Study the drawing (mm; zero at the part's minimum x, y, z) and answer. A direction names the side the tool comes from. Coordinates: 2 decimals unless noted, no trailing zeros. Order: outer loops, then holes, each group sorted by start corner. A loop starts at its lowest first (then second) coordinate and runs counter-clockwise, first axis right, second up.
1. Flat-ended cylindrical pins translate along their axes: pin 1 Ø6 at (x, z) = (38.5, 38.5) entering from -Y; pin 2 Ø4 at (y, z) = (7.5, 5) entering from -X; pin 3 Ø1.2 at (x, z) = (51.5, 2.5) entering from +Y; pin 4 Ø1.6 at (x, y) = (3.35, 15.2) entering from -Z. Find the tip coordinate at first contact, or state that the pin passes through.
2. Find the intervals of material crossed by probe 1 along Y at (x, z) = (53.25, 27.7); probe 2 along Z at (x, y) = (51, 9.5); probe 3 along Z at (x, y) = (42.5, 15.5), in increasing order.
3. The part is cut by section D-D, the plane y = 5.8. Give the vertices of the cut face in (x, z).
4. The part is cut by section B-B, the plane z = 27.5. Give the vertices of the cut face in (x, y), then the cut area to 3 significant figures.
5. Determine the mould class of the marked faces 1, 2 and 3 for opening direction Z: +Z half, -Z half, draft (parallel to the pull), parting line (faces both ways), or undercut.
6. The part is cut by section A-A, the plane x = 50. Give the vertices of the cut face in (y, z), then the cut area to 3 significant figures.
7. The part is cut by section C-C, the plane x = 38.2. Give the vertices of the cut face in (y, z).
8. A tool of negligible diameter and unlimited length cuts with its end or side. For the marked faces 4, 5, 6 and 7, from which of +Z, -Z, +X, -X, +Y, -Y can it reach the whole face along a straight path? Write none if from no direction.
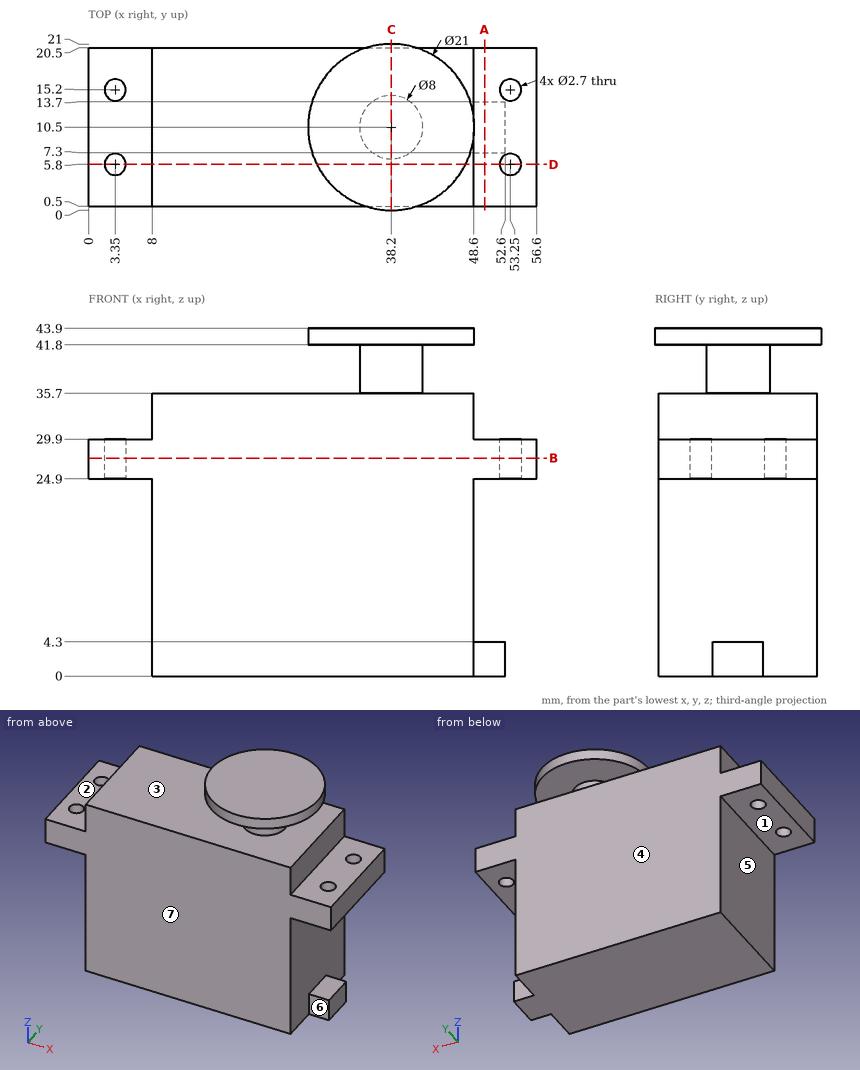
Geometry says:
1. pin 1: stops at y = 0.5
1. pin 2: stops at x = 8
1. pin 3: stops at y = 13.7
1. pin 4: passes through
2. probe 1: y = 0.5 to 4.45, 7.15 to 13.85, 16.55 to 20.5
2. probe 2: z = 0 to 4.3, 24.9 to 29.9
2. probe 3: z = 0 to 35.7, 41.8 to 43.9
3. outline: (0, 24.9) - (2, 24.9) - (2, 29.9) - (0, 29.9) - close; (4.7, 24.9) - (8, 24.9) - (8, 0) - (48.6, 0) - (48.6, 24.9) - (51.9, 24.9) - (51.9, 29.9) - (48.6, 29.9) - (48.6, 35.7) - (8, 35.7) - (8, 29.9) - (4.7, 29.9) - close; (28.81, 41.8) - (47.59, 41.8) - (47.59, 43.9) - (28.81, 43.9) - close; (54.6, 24.9) - (56.6, 24.9) - (56.6, 29.9) - (54.6, 29.9) - close
4. outline: (0, 0.5) - (56.6, 0.5) - (56.6, 20.5) - (0, 20.5) - close; hole circle Ø2.7 at (3.35, 5.8); hole circle Ø2.7 at (3.35, 15.2); hole circle Ø2.7 at (53.25, 5.8); hole circle Ø2.7 at (53.25, 15.2)
4. area: 1,110 mm2
5. face 1: -Z half
5. face 2: +Z half
5. face 3: undercut
6. outline: (0.5, 24.9) - (20.5, 24.9) - (20.5, 29.9) - (0.5, 29.9) - close; (7.3, 0) - (13.7, 0) - (13.7, 4.3) - (7.3, 4.3) - close
6. area: 128 mm2
7. outline: (0, 41.8) - (6.5, 41.8) - (6.5, 35.7) - (0.5, 35.7) - (0.5, 0) - (20.5, 0) - (20.5, 35.7) - (14.5, 35.7) - (14.5, 41.8) - (21, 41.8) - (21, 43.9) - (0, 43.9) - close
8. face 4: -Z, +X, -X, +Y
8. face 5: -Z, -X, +Y, -Y
8. face 6: -Z, +X, -Y
8. face 7: -Z, +X, -X, -Y
